Check sheet for the modelled part. Datum: model origin and axes. Units: mm. Round coordinates to 2 decimals unless told otherwise and drop trailing zeros. Use one line per item in the form item = value. Start each with the question number.
(1) Material ranges on probe 1 along X at (y, z) = (-304, 0.25); probe 2 along X at (y, z) = (-129.5, -6.5); probe 3 along Z at (x, y) = (20, -191), recorded low to high. Write a range as [from, to].
(2) Sectioned sample at A-A (y = -436.5). State how many separate pieces and enclosed holes the cut face has, and give its area (3 significant figures).
(3) Go/stop test with flat-tipped pins: pin 1 (6 mm diameter, centred on x = -20, y = -354.5, fed in from -Z); pin 2 (2 mm diameter, centred on y = -304.5, z = 3, fed in from -X); pin 3 (1.7 mm diameter, centred on x = -4, y = -187.5, fed in from +Z). Record where each tip stops, or that it passes through.
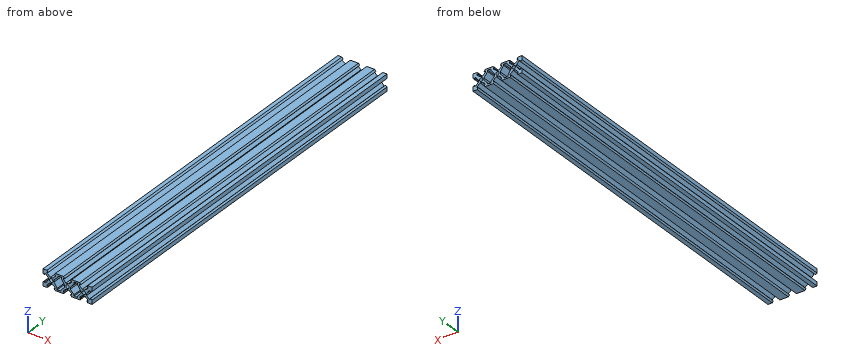
from build123d import *

# Parameters (mm, degrees)
F0_R     = 2.1
F0_W     = 2.608595
F0_H     = 1.64
F0_W_2   = 2.954579
F0_W_3   = 2.781998
F0_W_4   = 2.772428
F0_W_5   = 2.700623
F0_W_6   = 3.026465
F0_W_7   = 2.722846
F0_W_8   = 2.768436
F1_DEPTH = 500


with BuildPart() as f1:
    # F0 (on Front) → F1 (new body)
    with BuildSketch(Plane.XZ):
        Polygon((30, 4.805219), (30, 10), (24.818853, 10), (23.559123, 8.2), (24.85866, 8.2), (28.2, 8.2), (28.2, 4.872657), (28.2, 3.4364), align=None)
        Polygon((28.2, 8.2), (24.85866, 8.2), (24.85866, 6.56), (26.56, 6.56), (26.56, 4.872657), (28.2, 4.872657), align=None)
        Polygon((26.56, 6.56), (24.85866, 6.56), (20.776314, 3.45), (23.45, 3.45), (23.45, 0.429287), (26.56, 4.872657), align=None)
        Polygon((28.2, -5.054571), (26.56, -5.054571), (26.56, -6.56), (24.849551, -6.56), (24.849551, -8.2), (28.2, -8.2), align=None)
        Polygon((28.2, -3.583251), (28.2, -5.054571), (28.2, -8.2), (24.849551, -8.2), (23.522707, -8.2), (24.78151, -10), (30, -10), (30, -5.079649), align=None)
        Polygon((26.56, -5.054571), (23.45, -1.968018), (23.45, -3.45), (21.271573, -3.45), (24.849551, -6.56), (26.56, -6.56), align=None)
        Polygon((23.45, 3.45), (20.776314, 3.45), (18.152582, 3.45), (16.55, 3.45), (16.55, 0.581537), (16.55, -2.054411), (16.55, -3.45), (18.781548, -3.45), (21.271573, -3.45), (23.45, -3.45), (23.45, -1.968018), (23.45, 0.429287), align=None)
        with Locations((20, 0)):
            Circle(F0_R, mode=Mode.SUBTRACT)
        Polygon((16.55, 3.45), (18.152582, 3.45), (14.789955, 6.56), (12.18136, 6.56), (16.55, 0.581537), align=None)
        with Locations((13.485657, 7.38)):
            Rectangle(F0_W, F0_H)
        Polygon((12.18136, 8.2), (14.789955, 8.2), (16.369443, 8.2), (14.802462, 10), (5.216223, 10), (3.495616, 8.2), (5.084707, 8.2), (8.039286, 8.2), align=None)
        with Locations((6.561996, 7.38)):
            Rectangle(F0_W_2, F0_H)
        Polygon((3.45, 0.523604), (8.039286, 6.56), (5.084707, 6.56), (0.743741, 3.45), (3.45, 3.45), align=None)
        Polygon((16.55, -3.45), (16.55, -2.054411), (12.382907, -6.56), (15.164905, -6.56), (18.781548, -3.45), align=None)
        with Locations((13.773906, -7.38)):
            Rectangle(F0_W_3, F0_H)
        Polygon((15.164905, -8.2), (12.382907, -8.2), (7.965668, -8.2), (5.19324, -8.2), (3.534545, -8.2), (5.178779, -10), (15.299954, -10), (16.450917, -8.2), align=None)
        with Locations((6.579454, -7.38)):
            Rectangle(F0_W_4, F0_H)
        Polygon((5.19324, -6.56), (7.965668, -6.56), (3.45, -1.706813), (3.45, -3.45), (1.51754, -3.45), align=None)
        Polygon((3.45, -1.706813), (3.45, 0.523604), (3.45, 3.45), (0.743741, 3.45), (-1.908073, 3.45), (-3.45, 3.45), (-3.45, 0.529449), (-3.45, -2.140485), (-3.45, -3.45), (-1.461518, -3.45), (1.51754, -3.45), (3.45, -3.45), align=None)
        Circle(F0_R, mode=Mode.SUBTRACT)
        Polygon((-3.45, 3.45), (-1.908073, 3.45), (-4.804165, 6.56), (-7.504788, 6.56), (-3.45, 0.529449), align=None)
        with Locations((-6.154476, 7.38)):
            Rectangle(F0_W_5, F0_H)
        Polygon((-7.504788, 8.2), (-4.804165, 8.2), (-3.478876, 8.2), (-4.912788, 10), (-14.839575, 10), (-16.450822, 8.2), (-14.827697, 8.2), (-11.801232, 8.2), align=None)
        with Locations((-13.314464, 7.38)):
            Rectangle(F0_W_6, F0_H)
        Polygon((-16.55, 1.867669), (-11.801232, 6.56), (-14.827697, 6.56), (-17.999909, 3.45), (-16.55, 3.45), align=None)
        Polygon((-5.053682, -6.56), (-1.461518, -3.45), (-3.45, -3.45), (-3.45, -2.140485), (-7.776528, -6.56), align=None)
        with Locations((-6.415105, -7.38)):
            Rectangle(F0_W_7, F0_H)
        Polygon((-3.516317, -8.2), (-5.053682, -8.2), (-7.776528, -8.2), (-12.596157, -8.2), (-15.364593, -8.2), (-16.573226, -8.2), (-15.341443, -10), (-4.912339, -10), align=None)
        with Locations((-13.980375, -7.38)):
            Rectangle(F0_W_8, F0_H)
        Polygon((-15.364593, -6.56), (-12.596157, -6.56), (-16.55, -0.627868), (-16.55, -3.45), (-19.336489, -3.45), align=None)
        Polygon((-16.55, -0.627868), (-16.55, 1.867669), (-16.55, 3.45), (-17.999909, 3.45), (-20.69855, 3.45), (-23.45, 3.45), (-23.45, 2.055018), (-23.45, -0.513568), (-23.45, -3.45), (-21.768495, -3.45), (-19.336489, -3.45), (-16.55, -3.45), align=None)
        with Locations((-20, 0)):
            Circle(F0_R, mode=Mode.SUBTRACT)
        Polygon((-23.45, 3.45), (-20.69855, 3.45), (-25.162122, 6.56), (-26.56, 6.56), (-26.56, 5.223384), (-23.45, 2.055018), align=None)
        Polygon((-24.874446, -6.56), (-21.768495, -3.45), (-23.45, -3.45), (-23.45, -0.513568), (-26.56, -5.258857), (-26.56, -6.56), align=None)
        Polygon((-26.56, 6.56), (-25.162122, 6.56), (-25.162122, 8.2), (-28.2, 8.2), (-28.2, 5.223384), (-26.56, 5.223384), align=None)
        Polygon((-28.2, 8.2), (-25.162122, 8.2), (-23.471262, 8.2), (-25.197601, 10), (-30, 10), (-30, 5.174848), (-28.2, 3.632653), (-28.2, 5.223384), align=None)
        Polygon((-24.874446, -8.2), (-24.874446, -6.56), (-26.56, -6.56), (-26.56, -5.258857), (-28.2, -5.258857), (-28.2, -8.2), align=None)
        Polygon((-23.553334, -8.2), (-24.874446, -8.2), (-28.2, -8.2), (-28.2, -5.258857), (-28.2, -3.466297), (-30, -5.218167), (-30, -10), (-24.812492, -10), align=None)
    extrude(amount=F1_DEPTH)


solid = f1.part
Checks:
q1.probe_1 = [-23.45, -22.09], [-17.91, -16.55], [-3.45, -2.09], [2.09, 3.45], [16.55, 17.91], [22.09, 23.45]
q1.probe_2 = [-30, -24.81], [-15.44, -12.64], [-7.72, -4.98], [5.12, 7.91], [12.44, 15.23], [24.78, 30]
q1.probe_3 = [-3.45, -2.1], [2.1, 3.45]
q2.separate_pieces = 1
q2.enclosed_holes = 5
q2.area = 467 mm2
q3.pin_1 = -5.28
q3.pin_2 = -28.63
q3.pin_3 = 9.92
